from build123d import *

# Parameters (mm, degrees)
SKETCH1_W           = 1000
SKETCH1_H           = 1000
BOSS_EXTRUDE1_DEPTH = 30
SKETCH2_W           = 400
SKETCH2_H           = 300
CUT_EXTRUDE1_DEPTH  = 20
SKETCH3_W           = 400
SKETCH3_H           = 300
SKETCH3_W_2         = 360
SKETCH3_H_2         = 260
BOSS_EXTRUDE2_DEPTH = 10
CHAMFER1_SIZE       = 10
SKETCH5_W           = 490
SKETCH5_H           = 320
SKETCH5_W_2         = 940
SKETCH5_H_2         = 570
CUT_EXTRUDE2_DEPTH  = 10
BOSS_EXTRUDE5_DEPTH = 500
CHAMFER3_SIZE       = 10


with BuildPart() as part:
    # Sketch1 → Boss-Extrude1 (new body)
    with BuildSketch(Plane(origin=(0, 0, 0), x_dir=(1, 0, 0), z_dir=(0, 1, 0))):
        with Locations((500, -500)):
            Rectangle(SKETCH1_W, SKETCH1_H)
    extrude(amount=BOSS_EXTRUDE1_DEPTH)

    # Sketch2 → Cut-Extrude1 (cut)
    with BuildSketch(Plane(origin=(0, 30, 0), x_dir=(1, 0, 0), z_dir=(0, 1, 0))):
        with Locations((230, -200)):
            Rectangle(SKETCH2_W, SKETCH2_H)
    extrude(amount=-CUT_EXTRUDE1_DEPTH, mode=Mode.SUBTRACT)

    # Sketch3 → Boss-Extrude2 (add)
    with BuildSketch(Plane(origin=(0, 10, 0), x_dir=(1, 0, 0), z_dir=(0, 1, 0))):
        with Locations((230, -200)):
            Rectangle(SKETCH3_W, SKETCH3_H)
        with Locations((230, -200)):
            Rectangle(SKETCH3_W_2, SKETCH3_H_2, mode=Mode.SUBTRACT)
    extrude(amount=BOSS_EXTRUDE2_DEPTH)

    # Chamfer1
    chamfer1_edges = [part.edges().sort_by_distance(p)[0] for p in [
        (230, 10, 70),
        (410, 10, 200),
        (230, 10, 330),
        (50, 10, 200),
    ]]
    chamfer(chamfer1_edges, length=CHAMFER1_SIZE - 0.0001)  # a hair under: the kernel refuses the full size

    # Sketch5 → Cut-Extrude2 (cut)
    with BuildSketch(Plane(origin=(0, 30, 0), x_dir=(1, 0, 0), z_dir=(0, 1, 0))):
        with Locations((725, -190)):
            Rectangle(SKETCH5_W, SKETCH5_H)
        with Locations((500, -685)):
            Rectangle(SKETCH5_W_2, SKETCH5_H_2)
    extrude(amount=-CUT_EXTRUDE2_DEPTH, mode=Mode.SUBTRACT)

    # Sketch7 → Boss-Extrude5 (add)
    with BuildSketch(Plane(origin=(0, 20, 0), x_dir=(1, 0, 0), z_dir=(0, 1, 0))):
        Polygon((970, -400), (955, -400), (955, -955), (45, -955), (45, -400), (30, -400), (30, -970), (970, -970), align=None)
    extrude(amount=BOSS_EXTRUDE5_DEPTH)

    # Chamfer3
    chamfer3_edges = [part.edges().sort_by_distance(p)[0] for p in [
        (725, 20, 30),
        (970, 20, 190),
        (725, 20, 350),
        (480, 20, 190),
        (45, 20, 677.5),
        (500, 20, 400),
        (955, 20, 677.5),
        (500, 20, 955),
    ]]
    chamfer(chamfer3_edges, length=CHAMFER3_SIZE - 0.0001)  # a hair under: the kernel refuses the full size


solid = part.part
CAD build for the part. Positions are in the model's coordinates, mm. A direction names the side the tool comes from. Round coordinates to 2 decimals unless told otherwise and drop trailing zeros. Order: outer loops, then holes, each group sorted by start corner. A loop starts at its lowest first (then second) coordinate and runs counter-clockwise, first axis right, second up. Notation, with made-up numbers: (-20, 4.25) - (2, 4.25) arc R26 ccw to (2, 39.25) - close; hole circle Ø9 at (25, 45). An arc over 180 degrees is marked (long way). Return JSON: item names as keys, results as strings.
(1) Pin check, flat tips, straight feed: pin 1 Ø2 at (x, y) = (426, 168) entering from +Z; pin 2 Ø5 at (x, z) = (821, 352.5) entering from +Y; pin 3 Ø5 at (x, z) = (765, 814.5) entering from +Y. Stop position of each tip, or through.
Answer key:
{"pin 1": "stops at z = 970", "pin 2": "stops at y = 30", "pin 3": "stops at y = 20"}
(2) Pull direction Z, two halves, no side cores. Call faces 1 (the face through (1000, 15, 507)), 2 (the face through (493, 272, 970)), 3 (the face through (214, 20, 333)): +Z half, -Z half, draft (parallel to the pull), parting line (faces both ways), or undercut.
Answer key:
{"face 1": "draft", "face 2": "+Z half", "face 3": "undercut"}
(3) Cut at B-B (z = 775). Give the cut face in (x, y).
Answer key:
{"outline": "(0, 0) - (1000, 0) - (1000, 30) - (970, 30) - (970, 520) - (955, 520) - (955, 30) - (945, 20) - (55, 20) - (45, 30) - (45, 520) - (30, 520) - (30, 30) - (0, 30) - close"}
(4) Tool access for faces 4 (the face through (494, 20, 674)), 5 (the face through (30, 272, 681)), 6 (the face through (506, 272, 955)): list every direction of +Z, -Z, +X, -X, +Y, -Y with a clear straight run to the whole face (end or side of a thin tool).
Answer key:
{"face 4": "+Y", "face 5": "+Z, -Z, -X, +Y", "face 6": "-Z, +Y"}
(5) Cut at C-C (y = 172). Give the cut face in (x, z), then the cut area to 4 significant figures.
Answer key:
{"outline": "(30, 400) - (45, 400) - (45, 955) - (955, 955) - (955, 400) - (970, 400) - (970, 970) - (30, 970) - close", "area": "30,750 mm^2"}
(6) Wall check: probe 1 along X at (y, z) = (184, 545); probe 2 along Z at (x, y) = (283, 22.5); probe 3 along Z at (x, y) = (582.5, 27). Give the ranges that are in metal, low to high. Write a range as from..to.
Answer key:
{"probe 1": "x = 30..45, 955..970", "probe 2": "z = 0..50, 350..407.5, 947.5..1000", "probe 3": "z = 0..33, 347..403, 952..1000"}
